Part model, mm, in its own coordinate system. Face numbers are marked on the shaded views. Round coordinates to 2 decimals unless told otherwise and drop trailing zeros. Loops run counter-clockwise (first coordinate to the right, second up) from the corner with the lowest first, then second, coordinate; pieces in that order, holes last. Notation, with made-up numbers: M -39,-28 L -6,-28 A18 ccw -6,-9 Z; hole C 47,72.25 d6. An arc over 180 degrees is marked long. Answer as CSV lines item,"result". Start each with the question number.
Item 1: Band-saw the part on B-B (y = 42.5). Give the cut face in (x, z), and give its area (3 significant figures).
Item 2: Band-saw the part on D-D (x = 86.5). Give the cut face in (y, z), and give its area (3 significant figures).
Item 3: Band-saw the part on A-A (x = 9). Give the cut face in (y, z), and give its area (3 significant figures).
Item 4: Mould opens along X. For the marked faces 1, 2 and 3 say: pulls with the +X half, pulls with the -X half, needs draft (parallel to the pull), parting line crosses it, or undercut.
Item 5: Drop flat-ended pins along their axis: pin 1 Ø1.6 at (y, z) = (57.5, 21.5) entering from +X; pin 2 Ø1.5 at (x, y) = (-61.5, 108.5) entering from +Z; pin 3 Ø16.5 at (x, y) = (48, 86.5) entering from +Z; pin 4 Ø6.5 at (y, z) = (93, 12) entering from +X. Give the stop position or say it passes through.
Item 6: Band-saw the part on C-C (y = 206). Give the cut face in (x, z).
Item 7: Wall check: line 1 (Y direction, x = 3, z = 13.25); line 2 (X direction, y = 80.5, z = 5.5); line 3 (Y direction, x = -44, z = 1.75). Give the ranges that are in metal, low to high.
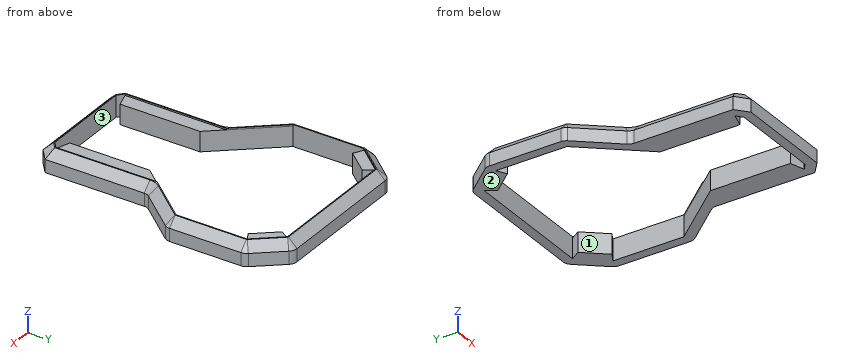
```python
from build123d import *

# Parameters (mm, degrees)
RESSALTO_EXTRUS_O1_DEPTH = 22.5
CHANFRO1_SIZE            = 9
CORTE_EXTRUS_O1_REACH    = 24.5
ESBO_O3_W                = 1139.230904301
ESBO_O3_H                = 709.798033895
CORTE_EXTRUS_O5_DEPTH    = 1.5
CORTE_EXTRUS_O6_REACH    = 23


with BuildPart() as part:
    # Esboço1 → Ressalto-extrusão1 (new body, symmetric)
    with BuildSketch(Plane.XY):
        with BuildLine():
            Line((-69.991831819, 290.260059805), (69.991831819, 290.260059805))
            ThreePointArc((69.991831819, 290.260059805), (74.218014437, 289.323137676), (77.652276251, 286.687935902))
            Line((77.652276251, 286.687935902), (100.660444431, 259.267868814))
            ThreePointArc((100.660444431, 259.267868814), (102.396926208, 256.26019415), (103, 252.839992717))
            Line((103, 252.839992717), (103, 177.526516487))
            ThreePointArc((103, 177.526516487), (102.453136861, 174.425101506), (100.878507208, 171.697762944))
            Line((100.878507208, 171.697762944), (67.121492792, 131.46771974))
            ThreePointArc((67.121492792, 131.46771974), (65.546863139, 128.740381178), (65, 125.638966197))
            Line((65, 125.638966197), (65, 20.90019601))
            Line((65, 20.90019601), (52.319579452, 10.260059805))
            Line((52.319579452, 10.260059805), (-52.319579452, 10.260059805))
            Line((-52.319579452, 10.260059805), (-65, 20.90019601))
            Line((-65, 20.90019601), (-65, 125.638966197))
            ThreePointArc((-65, 125.638966197), (-65.546863139, 128.740381178), (-67.121492792, 131.46771974))
            Line((-67.121492792, 131.46771974), (-100.878507208, 171.697762944))
            ThreePointArc((-100.878507208, 171.697762944), (-102.453136861, 174.425101506), (-103, 177.526516487))
            Line((-103, 177.526516487), (-103, 252.839992717))
            ThreePointArc((-103, 252.839992717), (-102.396926208, 256.26019415), (-100.660444431, 259.267868814))
            Line((-100.660444431, 259.267868814), (-77.652276251, 286.687935902))
            ThreePointArc((-77.652276251, 286.687935902), (-74.218014437, 289.323137676), (-69.991831819, 290.260059805))
        make_face()
        Polygon((-63.705668081, 270.260059805), (63.705668081, 270.260059805), (83, 247.265970424), (83, 181.505464287), (40, 130.260059805), (40, 30.260059805), (-40, 30.260059805), (-40, 130.260059805), (-83, 181.505464287), (-83, 247.265970424), align=None, mode=Mode.SUBTRACT)
    extrude(amount=RESSALTO_EXTRUS_O1_DEPTH, both=True)

    # Chanfro1
    chanfro1_edges = [part.edges().sort_by_distance(p)[0] for p in [
        (65, 73.269581104, 22.5),
        (65.546863139, 128.740381178, 22.5),
        (84, 151.582741342, 22.5),
        (102.453136861, 174.425101506, 22.5),
        (103, 215.183254602, 22.5),
        (102.396926208, 256.26019415, 22.5),
        (89.156360341, 272.977902358, 22.5),
        (74.218014437, 289.323137676, 22.5),
        (0, 290.260059805, 22.5),
        (-74.218014437, 289.323137676, 22.5),
        (-89.156360341, 272.977902358, 22.5),
        (-102.396926208, 256.26019415, 22.5),
        (-103, 215.183254602, 22.5),
        (-102.453136861, 174.425101506, 22.5),
        (-84, 151.582741342, 22.5),
        (-65.546863139, 128.740381178, 22.5),
        (-65, 73.269581104, 22.5),
        (-58.659789726, 15.580127908, 22.5),
        (0, 10.260059805, 22.5),
        (58.659789726, 15.580127908, 22.5),
    ]]
    chamfer(chanfro1_edges, length=CHANFRO1_SIZE)

    # Esboço3 → Corte-extrusão1 (cut, up to next)
    with BuildSketch(Plane.XY, mode=Mode.PRIVATE) as corte_extrus_o1_sk1:
        with Locations((-153.157436203, 152.53565808)):
            Rectangle(ESBO_O3_W, ESBO_O3_H)
    corte_extrus_o1_tool1 = extrude(corte_extrus_o1_sk1.sketch, amount=-CORTE_EXTRUS_O1_REACH, mode=Mode.PRIVATE) & part.part
    add(corte_extrus_o1_tool1.solids().sort_by_distance((-153.157436, 152.535658, 0))[0], mode=Mode.SUBTRACT)

    # Esboço4 → Corte-extrusão5 (cut)
    with BuildSketch(Plane.XY.offset(22.5)):
        Polygon((69.991831819, 280.260059805), (-69.991831819, 280.260059805), (-93, 252.839992717), (-93, 177.865761944), (-55, 132.579125426), (-55, 25.563272592), (-48.679877109, 20.260059805), (48.679877109, 20.260059805), (55, 25.563272592), (55, 132.579125426), (93, 177.865761944), (93, 252.839992717), align=None)
        Polygon((40, 30.260059805), (-40, 30.260059805), (-40, 130.260059805), (-83, 181.505464287), (-83, 247.265970424), (-63.705668081, 270.260059805), (63.705668081, 270.260059805), (83, 247.265970424), (83, 181.505464287), (40, 130.260059805), align=None, mode=Mode.SUBTRACT)
    extrude(amount=-CORTE_EXTRUS_O5_DEPTH, mode=Mode.SUBTRACT)

    # Esboço5 → Corte-extrusão6 (cut, up to next)
    with BuildSketch(Plane.XY.offset(21), mode=Mode.PRIVATE) as corte_extrus_o6_sk1:
        Polygon((-93, 252.839992717), (-83, 247.265970424), (-83, 181.505464287), (-40, 130.260059805), (-40, 114.702821537), (-93, 177.865761944), align=None)
    corte_extrus_o6_tool1 = extrude(corte_extrus_o6_sk1.sketch, amount=-CORTE_EXTRUS_O6_REACH, mode=Mode.PRIVATE) & part.part
    add(corte_extrus_o6_tool1.solids().sort_by_distance((-88.720359, 248.760631, 21))[0], mode=Mode.SUBTRACT)
    # Esboço5 → Corte-extrusão6 (cut, up to next)
    with BuildSketch(Plane.XY.offset(21), mode=Mode.PRIVATE) as corte_extrus_o6_sk2:
        Polygon((-63.705668081, 270.260059805), (-69.991831819, 280.260059805), (69.991831819, 280.260059805), (63.705668081, 270.260059805), align=None)
    corte_extrus_o6_tool2 = extrude(corte_extrus_o6_sk2.sketch, amount=-CORTE_EXTRUS_O6_REACH, mode=Mode.PRIVATE) & part.part
    add(corte_extrus_o6_tool2.solids().sort_by_distance((0, 275.338423, 21))[0], mode=Mode.SUBTRACT)
    # Esboço5 → Corte-extrusão6 (cut, up to next)
    with BuildSketch(Plane.XY.offset(21), mode=Mode.PRIVATE) as corte_extrus_o6_sk3:
        Polygon((-55, 25.563272592), (-40, 30.260059805), (40, 30.260059805), (55, 25.563272592), (48.679877109, 20.260059805), (-48.679877109, 20.260059805), align=None)
    corte_extrus_o6_tool3 = extrude(corte_extrus_o6_sk3.sketch, amount=-CORTE_EXTRUS_O6_REACH, mode=Mode.PRIVATE) & part.part
    add(corte_extrus_o6_tool3.solids().sort_by_distance((0, 25.125903, 21))[0], mode=Mode.SUBTRACT)
    # Esboço5 → Corte-extrusão6 (cut, up to next)
    with BuildSketch(Plane.XY.offset(21), mode=Mode.PRIVATE) as corte_extrus_o6_sk4:
        Polygon((40, 114.702821537), (93, 177.865761944), (93, 252.839992717), (83, 247.265970424), (83, 181.505464287), (40, 130.260059805), align=None)
    corte_extrus_o6_tool4 = extrude(corte_extrus_o6_sk4.sketch, amount=-CORTE_EXTRUS_O6_REACH, mode=Mode.PRIVATE) & part.part
    add(corte_extrus_o6_tool4.solids().sort_by_distance((65.366594, 147.235332, 21))[0], mode=Mode.SUBTRACT)


solid = part.part
```
Answer block:
1,outline,"M -65,0 L -40,0 L -40,21 L -55,21 L -55,22.5 L -56,22.5 L -65,13.5 Z; M 40,0 L 65,0 L 65,13.5 L 56,22.5 L 55,22.5 L 55,21 L 40,21 Z"
1,area,"999 mm^2"
2,outline,"M 154.56,0 L 170.12,0 L 170.12,22.5 L 168.56,22.5 L 154.56,13.5 Z; M 249.22,0 L 276.14,0 L 276.14,13.5 L 262.14,22.5 L 260.59,22.5 L 260.59,21 L 249.22,21 Z"
2,area,"813 mm^2"
3,outline,"M 10.26,0 L 20.26,0 L 20.26,22.5 L 19.26,22.5 L 10.26,13.5 Z; M 280.26,0 L 290.26,0 L 290.26,13.5 L 281.26,22.5 L 280.26,22.5 Z"
3,area,"369 mm^2"
4,face 1,"undercut"
4,face 2,"needs draft"
4,face 3,"undercut"
5,pin 1,"stops at x = 57.8"
5,pin 2,"stops at z = 17.75"
5,pin 3,"stops at z = 22.5"
5,pin 4,"stops at x = 65"
6,outline,"M -103,0 L -93,0 L -93,22.5 L -94,22.5 L -103,13.5 Z; M 93,0 L 103,0 L 103,13.5 L 94,22.5 L 93,22.5 Z"
7,line 1,"y = 10.26 to 20.26, 280.26 to 290.26"
7,line 2,"x = -65 to -40, 40 to 65"
7,line 3,"y = 10.26 to 20.26, 29.01 to 119.47, 280.26 to 290.26"
